```python
from build123d import *

# Parameters (mm, degrees)
F0_R     = 10.832434
F1_DEPTH = 68.66801
F2_R     = 4.08089
F3_DEPTH = 25.4
F4_W     = 14.424835
F4_H     = 4.475396
F5_DEPTH = 25.4


with BuildPart() as f1:
    # F0 (on Right) → F1 (new body)
    with BuildSketch(Plane.YZ):
        Circle(F0_R)
    extrude(amount=F1_DEPTH)

    # F2 (on face) → F3 (join)
    with BuildSketch(Plane.YZ.offset(68.66801)):
        Circle(F2_R)
    extrude(amount=F3_DEPTH)

    # F4 (on face) → F5 (cut)
    with BuildSketch(Plane(origin=(0, 0, 0), x_dir=(0, -1, 0), z_dir=(-1, 0, 0))):
        with Locations((-1.116385, -0.288975)):
            Rectangle(F4_W, F4_H)
    extrude(amount=-F5_DEPTH, mode=Mode.SUBTRACT)


solid = f1.part
```
Work out the finished part from the listing and answer in its coordinate system (mm). A direction names the side the tool comes from. Give positions to 0.01 mm unless a question says otherwise; leave off trailing zeros. Loops run counter-clockwise (first coordinate to the right, second up) from the corner with the lowest first, then second, coordinate; pieces in that order, holes last. Notation, with made-up numbers: (25.25, -7) - (44.25, -7) arc R25 cw to (44.25, 20) - close; hole circle Ø10 at (1.25, -14). An arc over 180 degrees is marked (long way). One line per question, with ' | ' between items.
(1) Straight lines are drawn through the part: probe 1 along Z at (x, y) = (25, 0.25); probe 2 along X at (y, z) = (9.5, -3); probe 3 along Z at (x, y) = (61, 5.25). For each, find the intervals that lie inside material, in ascending order.
Recorded:
probe 1: z = -10.83 to -2.53, 1.95 to 10.83 | probe 2: x = 0 to 68.67 | probe 3: z = -9.48 to 9.48
(2) The part is cut by section B-B (z = 0). Write down the section's boundary in (x, y), then the cut area to 3 significant figures.
Recorded:
outline: (0, -10.83) - (68.67, -10.83) - (68.67, -4.08) - (94.07, -4.08) - (94.07, 4.08) - (68.67, 4.08) - (68.67, 10.83) - (0, 10.83) - (0, 8.33) - (25.4, 8.33) - (25.4, -6.1) - (0, -6.1) - close | area: 1,330 mm²
(3) The part is cut by section D-D (z = 5.5). Write down the section's boundary in (x, y).
Recorded:
outline: (0, -9.33) - (68.67, -9.33) - (68.67, 9.33) - (0, 9.33) - close
(4) The part is cut by section A-A (y = 0). Write down the section's boundary in (x, z).
Recorded:
outline: (0, -10.83) - (68.67, -10.83) - (68.67, -4.08) - (94.07, -4.08) - (94.07, 4.08) - (68.67, 4.08) - (68.67, 10.83) - (0, 10.83) - (0, 1.95) - (25.4, 1.95) - (25.4, -2.53) - (0, -2.53) - close
(5) The part is cut by section C-C (x = 75). Write down the section's boundary in (y, z), then the cut area to 3 significant figures.
Recorded:
outline: circle Ø8.16 at (0, 0) | area: 52.3 mm²
(6) Each of these flat-tipped pins is pushed along its axis until it touches: pin 1 Ø8 at (x, y) = (78.5, -3) entering from -Z; pin 2 Ø6 at (x, y) = (66.5, 5.5) entering from -Z; pin 3 Ø2 at (x, z) = (7.5, 0.5) entering from +Y; pin 4 Ø1 at (y, z) = (-5.5, -8.5) entering from +X. Where does it stop, or does it pass through?
Recorded:
pin 1: stops at z = -4.08 | pin 2: stops at z = -10.54 | pin 3: stops at y = 10.83 | pin 4: stops at x = 68.67
(7) The mould has two halves that part along Y. Classify faces 4 (the face through (25.4, 1, 0)), 5 (the face through (81.19, -3.24, -2.48)), 6 (the face through (94.068, 0, 0)): +Y half, -Y half, draft (parallel to the pull), parting line (faces both ways), or undercut.
Recorded:
face 4: undercut | face 5: parting line | face 6: draft
(8) A tool of negligible diameter and unlimited length cuts with its end or side. For faces 1 (the face through (13, 1, 1.949)), 2 (the face through (68.668, 0, -5)), 3 (the face through (33.853, 10.332, 3.254)), from which of +Z, -Z, +X, -X, +Y, -Y can it reach the whole face along a straight path? Write none if from no direction.
Recorded:
face 1: -X | face 2: +X | face 3: +X, -X
